Read the model definition and answer for the solid it produces. Units are mm, in the model's axes. A direction names the side the tool comes from. Coordinates: 2 decimals unless noted, no trailing zeros. Write each loop counter-clockwise with the first axis right and the second up, starting at its lowest first coordinate (ties: lowest second). Pieces come first, ordered by that corner, then holes. Notation, with made-up numbers: (-36, 25.25) -> (-24, 25.25) arc R16 cw to (-24, 53.25) -> close; hole circle Ø3 at (75, 22.25). An arc over 180 degrees is marked (long way). Return JSON: item names as keys, results as strings.
from build123d import *

# Parameters (mm, degrees)
CHAMFER1_SIZE      = 4
SKETCH5_R          = 2.75
CUT_EXTRUDE4_DEPTH = 20
CUT_EXTRUDE5_DEPTH = 76.37904218
FILLET2_R          = 3
SKETCH7_R          = 42.25
CUT_EXTRUDE6_DEPTH = 2
SKETCH8_R          = 42.25
SKETCH8_R_2        = 40.25
CUT_EXTRUDE7_DEPTH = 4


with BuildPart() as part:
    # Sketch1 → Revolve1 (revolve)
    with BuildSketch(Plane(origin=(0, 0, 0), x_dir=(0, 0, -1), z_dir=(1, 0, 0)), mode=Mode.PRIVATE) as revolve1_sk:
        Polygon((5, 29), (5, 32), (15, 32), (15, 53), (7, 53), (7, 46), (4, 46), (4, 41), (1, 41), (1, 36), (0, 36), (0, 29), align=None)
    revolve(revolve1_sk.sketch.rotate(Axis((0, 0, 0), (0, 0, -1)), 90), axis=Axis((0, 0, 0), (0, 0, -1)))

    # Chamfer1
    chamfer1_edges = [part.edges().sort_by_distance(p)[0] for p in [
        (-29, 0, 0),
    ]]
    chamfer(chamfer1_edges, length=CHAMFER1_SIZE)

    # Sketch5 → Cut-Extrude4 (cut)
    with BuildSketch(Plane(origin=(0, 0, -15), x_dir=(-1, 0, 0), z_dir=(0, 0, -1))):
        with Locations((0, 47.5)):
            Circle(SKETCH5_R)
        with Locations((33.587572106, -33.587572106)):
            Circle(SKETCH5_R)
        with Locations((0, -47.5)):
            Circle(SKETCH5_R)
        with Locations((-33.587572106, 33.587572106)):
            Circle(SKETCH5_R)
    extrude(amount=-CUT_EXTRUDE4_DEPTH, mode=Mode.SUBTRACT)

    # Sketch6 → Cut-Extrude5 (cut, through all)
    with BuildSketch(Plane.XY.offset(-7)):
        with BuildLine():
            Line((26.571699547, 45.857875912), (23.865580267, 39.324726045))
            ThreePointArc((23.865580267, 39.324726045), (17.603437889, 42.498458496), (10.931266811, 44.682294098))
            Line((10.931266811, 44.682294098), (13.637386091, 51.215443966))
            ThreePointArc((13.637386091, 51.215443966), (20.282221915, 48.965615223), (26.571699547, 45.857875912))
        make_face()
    extrude(amount=-CUT_EXTRUDE5_DEPTH, mode=Mode.SUBTRACT)

    # Fillet2
    fillet2_edges = [part.edges().sort_by_distance(p)[0] for p in [
        (23.865580267, 39.324726045, -11),
        (10.931266811, 44.682294098, -11),
    ]]
    fillet(fillet2_edges, radius=FILLET2_R)

    # Sketch7 → Cut-Extrude6 (cut)
    with BuildSketch(Plane(origin=(0, 0, -15), x_dir=(-1, 0, 0), z_dir=(0, 0, -1))):
        Circle(SKETCH7_R)
    extrude(amount=-CUT_EXTRUDE6_DEPTH, mode=Mode.SUBTRACT)

    # Sketch8 → Cut-Extrude7 (cut)
    with BuildSketch(Plane(origin=(0, 0, -13), x_dir=(-1, 0, 0), z_dir=(0, 0, -1))):
        Circle(SKETCH8_R)
        Circle(SKETCH8_R_2, mode=Mode.SUBTRACT)
    extrude(amount=-CUT_EXTRUDE7_DEPTH, mode=Mode.SUBTRACT)


solid = part.part
1. The part is cut by section C-C (x = 0). Count the separate pieces of the cut face and the enclosed holes in it, then the cut area to 4 significant figures.
Taken from the geometry:
{"separate pieces": "4", "enclosed holes": "0", "area": "343.5 mm2"}
2. Flat-ended cylindrical pins translate along their axes: pin 1 Ø1 at (x, z) = (-19, -13) entering from -Y; pin 2 Ø2 at (y, z) = (27, -5) entering from +X; pin 3 Ø8 at (y, z) = (21, -2) entering from +X; pin 4 Ø3.5 at (x, y) = (0, 47.5) entering from +Z. Find the tip coordinate at first contact, or state that the pin passes through.
Taken from the geometry:
{"pin 1": "stops at y = -49.67", "pin 2": "stops at x = 37.95", "pin 3": "stops at x = 42.53", "pin 4": "passes through"}
3. For a pull along Y with two mould halves and no side action, classify faces 5 (the face through (-6.94, 31.24, -9.06)), 6 (the face through (-0.2, 36.3, -1)), 7 (the face through (25.874, 44.173, -10.944)) as +Y half, -Y half, draft (parallel to the pull), parting line (faces both ways), or undercut.
Taken from the geometry:
{"face 5": "undercut", "face 6": "draft", "face 7": "+Y half"}
4. Consider L1, parallel to Y at x = 0, z = -8.5; L2, parallel to Y at x = 0, z = -12.7; L3, parallel to Y at x = 33.5, z = -10.5. Determine where each line is inside the solid, lowest interval first.
Taken from the geometry:
{"L1": "y = -53 to -50.25, -44.75 to -32, 32 to 44.75, 50.25 to 53", "L2": "y = -53 to -50.25, -44.75 to -42.25, -40.25 to -32, 32 to 40.25, 42.25 to 44.75, 50.25 to 53", "L3": "y = -41.07 to -25.75, -22.31 to 22.31, 25.75 to 30.84, 36.34 to 41.07"}
5. A tool of negligible diameter and unlimited length cuts with its end or side. For faces 1 (the face through (12.286, 45.358, -11.056)), 2 (the face through (-42.77, 16.93, -5.48)), 3 (the face through (-7, 41, -4)), 4 (the face through (42.77, -16.93, -5.48)), from which of +Z, -Z, +X, -X, +Y, -Y can it reach the whole face along a straight path? Write none if from no direction.
Taken from the geometry:
{"face 1": "+Z, -Z", "face 2": "+Z, -X", "face 3": "+Z", "face 4": "+Z, +X"}
6. The part is cut by section D-D (y = -47.5). Determine the outline of the cut face in (x, z), then the cut area to 3 significant figures.
Taken from the geometry:
{"outline": "(-23.51, -15) -> (-2.75, -15) -> (-2.75, -7) -> (-23.51, -7) -> close; (2.75, -15) -> (23.51, -15) -> (23.51, -7) -> (2.75, -7) -> close", "area": "332 mm2"}
7. The part is cut by section B-B (z = -10.5). Determine the outline of the cut face in (x, y), then the cut area to 3 significant figures.
Taken from the geometry:
{"outline": "circle Ø80.5 at (0, 0); (12.22, 47.8) -> (13.64, 51.22) arc R53 ccw (long way) to (26.57, 45.86) -> (25.16, 42.44) arc R3 cw to (21.01, 40.92) arc R46 ccw to (14.08, 43.79) arc R3 cw to start; hole circle Ø84.5 at (0, 0); hole circle Ø5.5 at (-33.59, -33.59); hole circle Ø64 at (0, 0); hole circle Ø5.5 at (0, -47.5); hole circle Ø5.5 at (0, 47.5); hole circle Ø5.5 at (33.59, 33.59)", "area": "4,900 mm2"}
